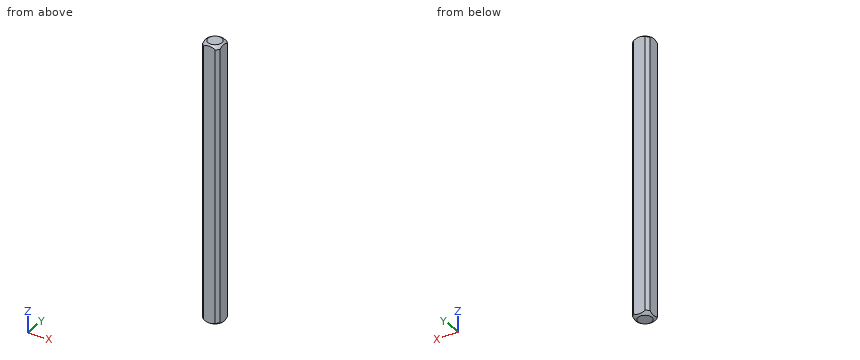
```python
from build123d import *

# Parameters (mm, degrees)
SKETCH1_W           = 6.35
SKETCH1_H           = 6.35
BOSS_EXTRUDE1_DEPTH = 50.8
SKETCH2_OUTSIDE_W   = 18.668
SKETCH2_OUTSIDE_H   = 18.668
SKETCH2_OUTSIDE_R   = 3.81
CUT_EXTRUDE1_DEPTH  = 51.8


with BuildPart() as part:
    # Sketch1 → Boss-Extrude1 (new body)
    with BuildSketch(Plane.XY):
        Rectangle(SKETCH1_W, SKETCH1_H)
    extrude(amount=BOSS_EXTRUDE1_DEPTH)

    # Sketch2 outside → Cut-Extrude1 (cut, through all)
    with BuildSketch(Plane(origin=(0, 0, 0), x_dir=(-1, 0, 0), z_dir=(0, 0, -1))):
        Rectangle(SKETCH2_OUTSIDE_W, SKETCH2_OUTSIDE_H)
        Circle(SKETCH2_OUTSIDE_R, mode=Mode.SUBTRACT)
    extrude(amount=-CUT_EXTRUDE1_DEPTH, mode=Mode.SUBTRACT)

    # Sketch3 → Cut-Revolve1 (revolve, cut)
    with BuildSketch(Plane(origin=(0, 0, 0), x_dir=(1, 0, 0), z_dir=(0, 1, 0))):
        with BuildLine():
            Line((-5.053685963, -3.893335876), (-5.053685963, 5.740530545))
            Line((-5.053685963, 5.740530545), (0, 5.740530545))
            Line((0, 5.740530545), (0, 0.670274551))
            ThreePointArc((0, 0.670274551), (-3.404639553, -0.639469554), (-5.053685963, -3.893335876))
        make_face()
    revolve(axis=Axis((0, 0, 50.8), (0, 0, -1)), mode=Mode.SUBTRACT)

    # Mirror1: part across plane


with BuildPart() as part_1:
    add(part.part)
    add(part.part.mirror(Plane(origin=(0, 0, 50.8), x_dir=(1, 0, 0), z_dir=(0, 0, -1))))


solid = part_1.part
```
CAD build for the part. Positions are in the model's coordinates, mm. Round coordinates to 2 decimals unless told otherwise and drop trailing zeros. Order: outer loops, then holes, each group sorted by start corner. A loop starts at its lowest first (then second) coordinate and runs counter-clockwise, first axis right, second up.
Q1. Slice it at A-A (z = 94.5). Write the cut outline in (x, y) (3 decimals).
Q2. Wall check: L1, parallel to Z at x = 2.5, y = 2; L2, parallel to Z at x = 0, y = 3; L3, parallel to Y at x = -2.25, z = 60.5. Give the ranges that are in metal, low to high.
Q3. Drop a flat-ended pin along its axis: pin 1 (3 mm diameter, centred on y = 2.5, z = 16, fed in from +X) (3 decimals). Give the stop position or say it passes through.
Results below:
1. outline: (-3.175, -2.106) arc R3.81 ccw to (-2.106, -3.175) - (2.106, -3.175) arc R3.81 ccw to (3.175, -2.106) - (3.175, 2.106) arc R3.81 ccw to (2.106, 3.175) - (-2.106, 3.175) arc R3.81 ccw to (-3.175, 2.106) - close
2. L1: z = 0.47 to 101.13
2. L2: z = 0.31 to 101.29
2. L3: y = -3.07 to 3.07
3. pin 1: stops at x = 3.175
